```python
from build123d import *

# Parameters (mm, degrees)
F0_W     = 161.6
F0_H     = 53.6
F0_W_2   = 78
F0_H_2   = 15.5
F0_W_3   = 65
F0_H_3   = 20
F1_DEPTH = 2
F2_D     = 5
F3_SIZE  = 1


with BuildPart() as f1:
    # F0 (on Top) → F1 (new body)
    with BuildSketch(Plane.XY):
        with Locations((0, -81.2946302295)):
            Rectangle(F0_W, F0_H)
        with BuildLine():
            ThreePointArc((-69.1, -100.4946302295), (-74.4, -95.1946302295), (-69.1, -89.8946302295))
            Line((-69.1, -89.8946302295), (-64.1, -89.8946302295))
            ThreePointArc((-64.1, -89.8946302295), (-58.8, -95.1946302295), (-64.1, -100.4946302295))
            Line((-64.1, -100.4946302295), (-69.1, -100.4946302295))
        make_face(mode=Mode.SUBTRACT)
        with BuildLine():
            ThreePointArc((-49, -100.4946302295), (-54.3, -95.1946302295), (-49, -89.8946302295))
            Line((-49, -89.8946302295), (-44, -89.8946302295))
            ThreePointArc((-44, -89.8946302295), (-38.7, -95.1946302295), (-44, -100.4946302295))
            Line((-44, -100.4946302295), (-49, -100.4946302295))
        make_face(mode=Mode.SUBTRACT)
        with BuildLine():
            ThreePointArc((-29.2, -100.4946302295), (-34.5, -95.1946302295), (-29.2, -89.8946302295))
            Line((-29.2, -89.8946302295), (-24.2, -89.8946302295))
            ThreePointArc((-24.2, -89.8946302295), (-18.9, -95.1946302295), (-24.2, -100.4946302295))
            Line((-24.2, -100.4946302295), (-29.2, -100.4946302295))
        make_face(mode=Mode.SUBTRACT)
        with BuildLine():
            ThreePointArc((-9.2, -100.4946302295), (-14.5, -95.1946302295), (-9.2, -89.8946302295))
            Line((-9.2, -89.8946302295), (-4.2, -89.8946302295))
            ThreePointArc((-4.2, -89.8946302295), (1.1, -95.1946302295), (-4.2, -100.4946302295))
            Line((-4.2, -100.4946302295), (-9.2, -100.4946302295))
        make_face(mode=Mode.SUBTRACT)
        with BuildLine():
            ThreePointArc((17.2, -100.4946302295), (11.9, -95.1946302295), (17.2, -89.8946302295))
            Line((17.2, -89.8946302295), (22.2, -89.8946302295))
            ThreePointArc((22.2, -89.8946302295), (27.5, -95.1946302295), (22.2, -100.4946302295))
            Line((22.2, -100.4946302295), (17.2, -100.4946302295))
        make_face(mode=Mode.SUBTRACT)
        with BuildLine():
            ThreePointArc((37.1, -100.4946302295), (31.8, -95.1946302295), (37.1, -89.8946302295))
            Line((37.1, -89.8946302295), (42.1, -89.8946302295))
            ThreePointArc((42.1, -89.8946302295), (47.4, -95.1946302295), (42.1, -100.4946302295))
            Line((42.1, -100.4946302295), (37.1, -100.4946302295))
        make_face(mode=Mode.SUBTRACT)
        with BuildLine():
            ThreePointArc((56.8, -100.4946302295), (51.5, -95.1946302295), (56.8, -89.8946302295))
            Line((56.8, -89.8946302295), (61.8, -89.8946302295))
            ThreePointArc((61.8, -89.8946302295), (67.1, -95.1946302295), (61.8, -100.4946302295))
            Line((61.8, -100.4946302295), (56.8, -100.4946302295))
        make_face(mode=Mode.SUBTRACT)
        with Locations((-39.8, -72.0446302295)):
            Rectangle(F0_W_2, F0_H_2, mode=Mode.SUBTRACT)
        with Locations((39.5, -73.2946302295)):
            Rectangle(F0_W_3, F0_H_3, mode=Mode.SUBTRACT)
    extrude(amount=F1_DEPTH)

    # F2 (through all)
    with Locations(Plane(origin=(0, 0, 0), x_dir=(1, 0, 0), z_dir=(0, 0, -1))):
        with Locations((-75, 60.2946302295), (-50, 60.2946302295), (-25, 60.2946302295)):
            Hole(F2_D / 2)

    # F3
    f3_edges = [f1.edges().sort_by_distance(p)[0] for p in [
        (-80.8, -81.29463, 2),
        (0, -108.09463, 2),
        (0, -54.49463, 2),
        (80.8, -81.29463, 2),
    ]]
    chamfer(f3_edges, length=F3_SIZE)


solid = f1.part
```
CAD build for the part. Positions are in the model's coordinates, mm. A direction names the side the tool comes from. Coordinates: 2 decimals unless noted, no trailing zeros. Order: outer loops, then holes, each group sorted by start corner. A loop starts at its lowest first (then second) coordinate and runs counter-clockwise, first axis right, second up. Notation, with made-up numbers: (49, 7) - (106, 7) arc R16 ccw to (106, 18) - close; hole circle Ø7 at (15.5, 14.25). An arc over 180 degrees is marked (long way). Use a Markdown table: item, result. Add a question column.
(1) Drill centre lines: line 1 along Y through (x, z) = (-7.5, 0.85); line 2 along Y through (x, z) = (-25, 0.8); line 3 along X through (y, z) = (-68, 0.3). Where is each one in solid material? Low to high. Write a range as [from, to].
(2) Saw through at B-B (z = 1.65). Count the separate pieces of the cut face and the enclosed holes in it, then the cut area to 3 significant figures.
(3) Which spindle directions (+Z, -Z, +X, -X, +Y, -Y) get a long thin tool onto all of the face, cutting with end or side? Do faces 3 (the face through (67.1, -95.1, 1)), 4 (the face through (-1, -81, 0)). Say none if no direction does.
(4) Pull direction Y, two halves, no side cores. Call faces 1 (the face through (-58.8, -95.1, 1)), 2 (the face through (-1, -81, 2)): +Y half, -Y half, draft (parallel to the pull), parting line (faces both ways), or undercut.
(5) Saw through at A-A (y = -77). Give the cut face in (x, z), then the cut area to 3 significant figures.
Solved:
| question | item | result |
|---|---|---|
| 1 | line 1 | y = [-108.09, -100.49], [-89.89, -79.79], [-64.29, -54.49] |
| 1 | line 2 | y = [-108.09, -100.49], [-89.89, -79.79], [-64.29, -62.79], [-57.79, -54.49] |
| 1 | line 3 | x = [-80.8, -78.8], [-0.8, 7], [72, 80.8] |
| 2 | separate pieces | 1 |
| 2 | enclosed holes | 12 |
| 2 | area | 4,830 mm² |
| 3 | face 3 | +Z, -Z |
| 3 | face 4 | -Z, +X, -X, +Y, -Y |
| 4 | face 1 | undercut |
| 4 | face 2 | draft |
| 5 | outline | (-80.8, 0) - (-78.8, 0) - (-78.8, 2) - (-79.8, 2) - (-80.8, 1) - close; (-0.8, 0) - (7, 0) - (7, 2) - (-0.8, 2) - close; (72, 0) - (80.8, 0) - (80.8, 1) - (79.8, 2) - (72, 2) - close |
| 5 | area | 36.2 mm² |
